```python
from build123d import *

# Parameters (mm, degrees)
EXTRUDE_1_DEPTH     = 67
SKETCH_2_R          = 5
CUT_EXTRUDE_1_DEPTH = 15
CUT_EXTRUDE_2_DEPTH = 3
SKETCH_4_R          = 7
SKETCH_4_R_2        = 5
EXTRUDE_2_DEPTH     = 5
SKETCH_5_R          = 3.5
CUT_EXTRUDE_4_DEPTH = 10


with BuildPart() as part:
    # 草图1 → 凸台-拉伸1 (new body)
    with BuildSketch(Plane.XY):
        Polygon((8, 0), (-8, 0), (-6, 35), (6, 35), align=None)
    extrude(amount=EXTRUDE_1_DEPTH)

    # 草图2 → 切除-拉伸1 (cut, symmetric)
    with BuildSketch(Plane(origin=(0, 0, 0), x_dir=(0, 0, -1), z_dir=(1, 0, 0))):
        with BuildLine():
            Line((-67, 35), (-67, 6))
            Line((-67, 6), (-51.25, 6))
            Line((-51.25, 6), (-51.25, 17.25))
            ThreePointArc((-51.25, 17.25), (-46.051145366, 29.801145366), (-33.5, 35))
            Line((-33.5, 35), (-67, 35))
        make_face()
        with BuildLine():
            Line((0, 35), (-33.5, 35))
            ThreePointArc((-33.5, 35), (-20.948854634, 29.801145366), (-15.75, 17.25))
            Line((-15.75, 17.25), (-15.75, 6))
            Line((-15.75, 6), (0, 6))
            Line((0, 6), (0, 35))
        make_face()
        with Locations((-33.5, 17.25)):
            Circle(SKETCH_2_R)
    extrude(amount=CUT_EXTRUDE_1_DEPTH, both=True, mode=Mode.SUBTRACT)

    # 草图3 → 切除-拉伸2 (cut)
    with BuildSketch(Plane(origin=(8, 0, 0), x_dir=(0, 0, -1), z_dir=(1, 0, 0))):
        with BuildLine():
            Line((-49.25, 6), (-49.25, 0))
            Line((-49.25, 0), (-17.75, 0))
            Line((-17.75, 0), (-17.75, 6))
            Line((-17.75, 6), (-17.75, 17.25))
            ThreePointArc((-17.75, 17.25), (-33.5, 33), (-49.25, 17.25))
            Line((-49.25, 17.25), (-49.25, 6))
        make_face()
    cut_extrude_2 = extrude(amount=-CUT_EXTRUDE_2_DEPTH, mode=Mode.SUBTRACT)

    # 镜向1: 切除-拉伸2 across plane
    add(cut_extrude_2.mirror(Plane(origin=(0, 0, 0), x_dir=(0, 0, 1), z_dir=(1, 0, 0))), mode=Mode.SUBTRACT)

    # 草图4 → 凸台-拉伸2 (add)
    with BuildSketch(Plane(origin=(-10, 0, 0), x_dir=(0, 0, -1), z_dir=(1, 0, 0))):
        with Locations((-33.5, 17.25)):
            Circle(SKETCH_4_R)
        with Locations((-33.5, 17.25)):
            Circle(SKETCH_4_R_2, mode=Mode.SUBTRACT)
    extrude(amount=EXTRUDE_2_DEPTH)

    # 草图5 → 切除-拉伸4 (cut)
    with BuildSketch(Plane.XZ):
        with Locations((0, 60)):
            Circle(SKETCH_5_R)
        with Locations((0, 7)):
            Circle(SKETCH_5_R)
    extrude(amount=-CUT_EXTRUDE_4_DEPTH, mode=Mode.SUBTRACT)


solid = part.part
```
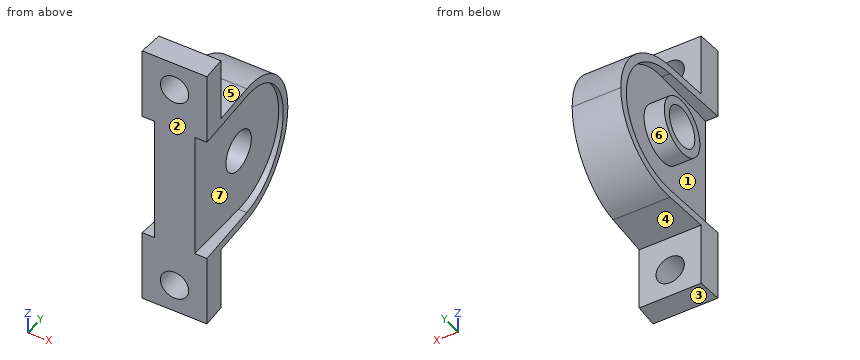
Work out the finished part from the listing and answer in its coordinate system (mm). Face numbers are marked on the shaded views. A direction names the side the tool comes from. Coordinates: 2 decimals unless noted, no trailing zeros. Loops run counter-clockwise (first coordinate to the right, second up) from the corner with the lowest first, then second, coordinate; pieces in that order, holes last. Notation, with made-up numbers: (15.5, -29) - (33.5, -29) arc R11 cw to (33.5, -20) - close; hole circle Ø9 at (-25.5, 5). An arc over 180 degrees is marked (long way). Use a Markdown table: item, result.
Item 1: Find section A-A, the plane x = 0. Determine the outline of the cut face in (y, z), and give its area (3 significant figures).
Evaluation:
| item | result |
|---|---|
| outline | (0, 0) - (6, 0) - (6, 3.5) - (0, 3.5) - close; (0, 10.5) - (6, 10.5) - (6, 15.75) - (17.25, 15.75) arc R17.75 ccw to (17.25, 51.25) - (6, 51.25) - (6, 56.5) - (0, 56.5) - close; (0, 63.5) - (6, 63.5) - (6, 67) - (0, 67) - close; hole circle Ø10 at (17.25, 33.5) |
| area | 1,130 mm2 |
Item 2: Given pin 1 Ø9 at (x, y) = (-3, 14) entering from -Z; pin 2 Ø11.5 at (y, z) = (17.25, 33.5) entering from +X; pin 3 Ø5.5 at (x, y) = (1, 10) entering from +Z; pin 4 Ø10 at (y, z) = (13, 58.5) entering from -X, each flat-ended and moving along its own axis, determine where each tip first touches the part or whether it passes through.
Evaluation:
| item | result |
|---|---|
| pin 1 | stops at z = 15.75 |
| pin 2 | stops at x = 5 |
| pin 3 | stops at z = 51.25 |
| pin 4 | passes through |
Item 3: Find section B-B, the plane z = 7. Determine the outline of the cut face in (x, y).
Evaluation:
| item | result |
|---|---|
| outline | (-8, 0) - (-3.5, 0) - (-3.5, 6) - (-7.66, 6) - close; (3.5, 0) - (8, 0) - (7.66, 6) - (3.5, 6) - close |
Item 4: Find section D-D, the plane y = 4. Determine the outline of the cut face in (x, z), and give its area (3 significant figures).
Evaluation:
| item | result |
|---|---|
| outline | (-7.77, 0) - (7.77, 0) - (7.77, 17.75) - (5, 17.75) - (5, 49.25) - (7.77, 49.25) - (7.77, 67) - (-7.77, 67) - (-7.77, 49.25) - (-5, 49.25) - (-5, 17.75) - (-7.77, 17.75) - close; hole circle Ø7 at (0, 7); hole circle Ø7 at (0, 60) |
| area | 790 mm2 |
Item 5: For the marked faces 4, 5, 6 and 7, determine the directions among +Z, -Z, +X, -X, +Y, -Y from which every point of the face is accessible in a straight line to the end or side of a thin tool.
Evaluation:
| item | result |
|---|---|
| face 4 | -Z, +X, -X, +Y |
| face 5 | +Z, +X, -X, +Y |
| face 6 | -X |
| face 7 | +X, -Y |
Item 6: Consider probe 1 along Z at (x, y) = (0, 4); probe 2 along Y at (x, z) = (-3, 33.5); probe 3 along Z at (x, y) = (-5.75, 6.5). Determine where each line is inside the solid, lowest interval first. Write a range as from..to.
Evaluation:
| item | result |
|---|---|
| probe 1 | z = 0..3.5, 10.5..56.5, 63.5..67 |
| probe 2 | y = 0..12.25, 22.25..35 |
| probe 3 | z = 15.75..17.75, 49.25..51.25 |
Item 7: Find section C-C, the plane y = 16.5. Determine the outline of the cut face in (x, z), and give its area (3 significant figures).
Evaluation:
| item | result |
|---|---|
| outline | (-10, 26.54) - (-5, 26.54) - (-5, 17.75) - (-7.06, 17.75) - (-7.06, 15.75) - (7.06, 15.75) - (7.06, 17.75) - (5, 17.75) - (5, 28.56) - (-10, 28.56) - close; (-10, 38.44) - (5, 38.44) - (5, 49.25) - (7.06, 49.25) - (7.06, 51.25) - (-7.06, 51.25) - (-7.06, 49.25) - (-5, 49.25) - (-5, 40.46) - (-10, 40.46) - close |
| area | 293 mm2 |
Item 8: The mould has two halves that part along Y. Classify the marked faces 1, 2 and 3: +Y half, -Y half, draft (parallel to the pull), parting line (faces both ways), or undercut.
Evaluation:
| item | result |
|---|---|
| face 1 | undercut |
| face 2 | -Y half |
| face 3 | draft |
